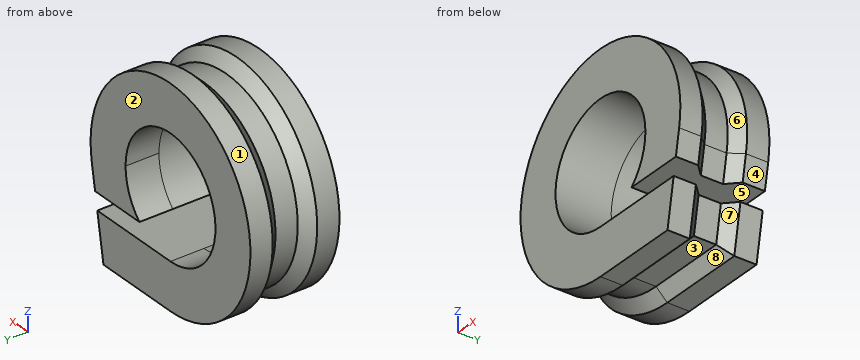
from build123d import *

# Parameters (mm, degrees)
BOSS_EXTRUDE1_DEPTH = 3
CHAMFER1_SIZE       = 1
BOSS_EXTRUDE2_DEPTH = 1


with BuildPart() as part:
    # Sketch1 → Boss-Extrude1 (new body)
    with BuildSketch(Plane(origin=(0, 0, 0), x_dir=(1, 0, 0), z_dir=(0, 1, 0))):
        with BuildLine():
            Line((8.055356459, 9.6), (0, 9.6))
            ThreePointArc((0, 9.6), (-6.170761053, -7.354026654), (9.454154429, 1.667022506))
            Line((9.454154429, 1.667022506), (9.060420249, 3.9))
            Line((9.060420249, 3.9), (3.734969879, 3.9))
            ThreePointArc((3.734969879, 3.9), (4.96632849, 2.120278596), (5.4, 0))
            ThreePointArc((5.4, 0), (-3.818376618, -3.818376618), (0, 5.4))
            Line((0, 5.4), (8.795929778, 5.4))
            Line((8.795929778, 5.4), (8.055356459, 9.6))
        make_face()
    extrude(amount=BOSS_EXTRUDE1_DEPTH)

    # Chamfer1
    chamfer1_edges = [part.edges().sort_by_distance(p)[0] for p in [
        (-6.170761053, 3, 7.354026654),
        (9.257287339, 3, -2.783511253),
        (8.425643119, 3, -7.5),
        (4.02767823, 3, -9.6),
    ]]
    chamfer(chamfer1_edges, length=CHAMFER1_SIZE)

    # Sketch3 → Boss-Extrude2 (add)
    with BuildSketch(Plane(origin=(0, 3, 0), x_dir=(1, 0, 0), z_dir=(0, 1, 0))):
        with BuildLine():
            Line((0, 5.4), (7.780503166, 5.4))
            Line((7.780503166, 5.4), (7.216256828, 8.6))
            Line((7.216256828, 8.6), (0, 8.6))
            ThreePointArc((0, 8.6), (-5.527973443, -6.587982211), (8.469346676, 1.493374328))
            Line((8.469346676, 1.493374328), (8.044993637, 3.9))
            Line((8.044993637, 3.9), (3.734969879, 3.9))
            ThreePointArc((3.734969879, 3.9), (-2.01246118, -5.010987927), (0, 5.4))
        make_face()
    extrude(amount=BOSS_EXTRUDE2_DEPTH)

    # Mirror1: part across plane


with BuildPart() as part_1:
    add(part.part)
    add(part.part.mirror(Plane.ZX.offset(4)))


solid = part_1.part
Can you work these out from the model? Positions are in its coordinate system, mm. Face numbers are marked on the shaded views. A direction names the side the tool comes from. Round coordinates to 2 decimals unless told otherwise and drop trailing zeros. Order: outer loops, then holes, each group sorted by start corner. A loop starts at its lowest first (then second) coordinate and runs counter-clockwise, first axis right, second up. Notation, with made-up numbers: (-38.5, 9.25) -> (-13.5, 9.25) arc R19 cw to (-13.5, 31.25) -> close; hole circle Ø6 at (51.5, -28). An arc over 180 degrees is marked (long way). Write each question's results on one line, items separated by ' | '. Start each with the question number.
Item 1: Please list where these lines run through material, in increasing order: L1, parallel to X at y = 6.35, z = 0; L2, parallel to Z at x = 0, y = 4.
Item 2: If we section it at B-B, the plane y = 1: Write out the boundary of the cut face in (x, z), then the cut area to 3 significant figures.
Item 3: If we section it at A-A, the plane y = 3.75: Write out the boundary of the cut face in (x, z) (1 decimal).
Item 4: If we section it at C-C, the plane x = 4.75: State how many separate pieces and enclosed holes the cut face has, then the cut area to 3 significant figures.
Item 5: Will these pins go through, and if not, where does the flat tip stop? pin 1 (9.5 mm diameter, centred on x = 0, z = 0, fed in from -Y); pin 2 (1 mm diameter, centred on y = 4, z = 3.5, fed in from -X); pin 3 (0.6 mm diameter, centred on x = 3.5, y = 3.5, fed in from -Z); pin 4 (2 mm diameter, centred on x = 7.5, y = 4.5, fed in from -Z).
Item 6: Which directions (+Z, -Z, +X, -X, +Y, -Y) give clear straight access to the entire face, cutting with the end or side of a thin tool? Please do the marked faces 4, 5, 6, 7 and 8.
Item 7: Thinking about a two-plate mould opening in Y: for the marked faces 1, 2 and 3, which applies, +Y half, -Y half, draft (parallel to the pull), parting line (faces both ways), or undercut?
Results:
1) L1: x = -9.6 to -5.4, 5.4 to 9.6 | L2: z = -8.6 to -5.4, 5.4 to 8.6
2) outline: (0, -9.6) -> (8.06, -9.6) -> (8.8, -5.4) -> (0, -5.4) arc R5.4 cw (long way) to (3.73, -3.9) -> (9.06, -3.9) -> (9.45, -1.67) arc R9.6 ccw (long way) to start | area: 201 mm2
3) outline: (0, -8.6) -> (7.2, -8.6) -> (7.8, -5.4) -> (0, -5.4) arc R5.4 cw (long way) to (3.7, -3.9) -> (8, -3.9) -> (8.5, -1.5) arc R8.6 ccw (long way) to start
4) separate pieces: 3 | enclosed holes: 0 | area: 83.9 mm2
5) pin 1: passes through | pin 2: stops at x = -8.06 | pin 3: stops at z = -8.6 | pin 4: stops at z = -9.1
6) face 4: -Z, +X, +Y, -Y | face 5: +X, +Y, -Y | face 6: none | face 7: -Z, +X | face 8: -Z, +X, -X
7) face 1: draft | face 2: +Y half | face 3: undercut
